Here's how the part is built. I have some questions about the finished solid (model axes, mm). Face numbers are marked on the shaded views. A direction names the side the tool comes from. Round coordinates to 2 decimals unless told otherwise and drop trailing zeros. Loops run counter-clockwise (first coordinate to the right, second up) from the corner with the lowest first, then second, coordinate; pieces in that order, holes last. Notation, with made-up numbers: M 74,42.5 L 98,42.5 A10 ccw 98,54.5 Z; hole C 0.25,-36.75 d8. An arc over 180 degrees is marked long. Use a Markdown table: item, result.
Autodesk Inventor part; units mm, degrees
ref_plane "Work Plane1" through (0, 0, -52.5) normal (0, 0, -1) x (-1, 0, 0)
ref_plane "YZ Plane" through (0, 0, 0) normal (1, 0, 0) x (0, 1, 0)
ref_plane "XZ Plane" through (0, 0, 0) normal (0, 1, 0) x (-1, 0, 0)
sketch "Sketch1" plane through (0, 0, 0) normal (0, 1, 0) x (-1, 0, 0)
  line L0 (0, 0) -> (105, 0)
  line L1 (105, 0) -> (105, -105)
  line L2 (105, -105) -> (0, -105)
  line L3 (0, -105) -> (0, 0)
  circle A0 centre (52.5, -52.5) radius 36.5
  dimension "d0" = 105
  dimension "d1" = 105
  dimension "d2" = 52.5
  dimension "d3" = 52.5
  dimension "d4" = 73
extrude "Extrusion1" add sketch "Sketch1" along normal blind 7
sketch "Sketch3" plane through (-105, 0, 0) normal (0, 0, 1) x (1, 0, 0)
  line L0 (105, 7) -> (0, 7)
  line L1 (0, 7) -> (105, 7)
  line L2 (105, 7) -> (105, -105)
  line L3 (105, -105) -> (0, -105)
  line L4 (0, -105) -> (0, 7)
  line L5 (0, 0) -> (105, 0)
  dimension "d7" = 105
extrude "Extrusion2" add sketch "Sketch3" along normal blind 5
sketch "Sketch4" plane through (-105, 0, -105) normal (-1, 0, 0) x (0, 0, 1)
  line L0 (0, 0) -> (0, 7)
  line L1 (0, 7) -> (110, 7)
  line L2 (110, 7) -> (110, -105)
  line L3 (110, -105) -> (0, -105)
  line L4 (0, -105) -> (0, 7)
  point P0 (105, 0)
extrude "Extrusion3" add sketch "Sketch4" along normal blind 5
sketch "Sketch6" plane through (0, 0, -105) normal (0, 0, -1) x (-1, 0, 0)
  line L0 (0, 7) -> (110, 7)
  line L1 (110, -105) -> (110, 7)
  line L2 (0, 7) -> (110, 7)
  line L3 (110, 7) -> (110, -105)
  line L4 (110, -105) -> (0, -105)
  line L5 (0, -105) -> (0, 7)
  point P0 (0, 0)
extrude "Extrusion4" add sketch "Sketch6" along normal blind 5
sketch "Sketch7" plane through (0, -105, 0) normal (1, 0, 0) x (0, 0, -1)
  line L0 (-5, 0) -> (-5, 112)
  line L1 (105, 0) -> (110, 0)
  line L2 (-5, 112) -> (110, 112)
  line L3 (110, 112) -> (110, 0)
  line L4 (110, 0) -> (-5, 0)
  line L5 (-5, 0) -> (-5, 112)
  point P0 (0, 105)
extrude "Extrusion5" add sketch "Sketch7" along normal blind 5
sketch "Sketch8" plane through (-110, -105, -110) normal (0, -1, 0) x (1, 0, 0)
  line L0 (0, 115) -> (115, 115)
  line L1 (0, 0) -> (115, 0)
  line L2 (0, 115) -> (115, 115)
  line L3 (115, 115) -> (115, 0)
  line L4 (115, 0) -> (0, 0)
  line L5 (0, 0) -> (0, 115)
  point P0 (110, 110)
extrude "Extrusion6" add sketch "Sketch8" along normal blind 5
sketch "Sketch9" plane through (0, 7, 0) normal (0, 1, 0) x (1, 0, 0)
  line L0 (-110, -5) -> (-110, 110)
  line L1 (-110, -5) -> (5, -5)
  line L2 (5, 110) -> (5, -5)
  line L3 (-110, 110) -> (5, 110)
  circle A0 centre (-52.5, 52.5) radius 36.5
  line L4 (-110, -5) -> (-110, 110)
  line L5 (-110, 110) -> (5, 110)
  line L6 (-110, -5) -> (5, -5)
  line L7 (5, -5) -> (5, 110)
  line L8 (5, 110) -> (-110, 110)
  line L9 (-110, 110) -> (-110, -5)
  circle A1 centre (-52.5, 52.5) radius 45
  dimension "d18" = 90
extrude "Extrusion7" add sketch "Sketch9" along normal blind 8 contours L0 L3 L2 L1
sketch "Sketch10" plane through (-52.5, 7, -52.5) normal (0, 1, 0) x (1, 0, 0)
  line L0 (57.5, -57.5) -> (-57.5, -57.5) construction
  line L1 (57.5, 57.5) -> (57.5, -57.5) construction
  line L2 (-57.5, -57.5) -> (57.5, 57.5) construction
  line L3 (57.5, 57.5) -> (-57.5, 57.5) construction
  line L4 (-57.5, 57.5) -> (57.5, -57.5) construction
  circle A0 centre (0, 0) radius 41.75 construction
  circle A1 centre (-29.5217, -29.5217) radius 1.9
  circle A2 centre (-29.5217, 29.5217) radius 1.9
  circle A3 centre (29.5217, 29.5217) radius 1.9
  circle A4 centre (29.5217, -29.5217) radius 1.9
  line L5 (0, -57.5) -> (0, 57.5) construction
  point P0 (52.5, -52.5)
  dimension "d21" = 3.8
  dimension "d22" = 83.5
  dimension "d23" = 3.8
  dimension "d24" = 3.8
  dimension "d25" = 3.8
  dimension "d26" = 45
extrude "Extrusion8" cut sketch "Sketch10" against normal blind 5
ref_plane "Work Plane1" through (0, 0, -52.5) normal (0, 0, -1) x (-1, 0, 0)
split "Split2" [suppressed]
chamfer "Chamfer1" distance 2 angle 45 1 edges at (-97.5, 15, -52.5)
sketch "Sketch15" plane through (0, 0, -52.5) normal (0, 0, -1) x (-1, 0, 0)
  line L0 (105, 14) -> (99.9142, 14)
  line L1 (99.9142, 14) -> (98.5, 12.5858)
  line L2 (98.5, 12.5858) -> (98.5, 6)
  line L3 (98.5, 6) -> (90, 6)
  line L4 (90, 6) -> (90, 1)
  line L5 (90, 1) -> (100, 1)
  arc A0 (106, -5) -> (100, 1) centre (100, -5) ccw
  line L6 (106, -5) -> (106, -100)
  arc A1 (100, -106) -> (106, -100) centre (100, -100) ccw
  line L7 (100, -106) -> (5, -106)
  arc A2 (-1, -100) -> (5, -106) centre (5, -100) ccw
  line L8 (-1, -100) -> (-1, -5)
  arc A3 (5, 1) -> (-1, -5) centre (5, -5) ccw
  line L9 (5, 1) -> (15, 1)
  line L10 (15, 1) -> (15, 6)
  line L11 (15, 6) -> (6.5, 6)
  line L12 (6.5, 6) -> (6.5, 12.5858)
  line L13 (6.5, 12.5858) -> (5.0858, 14)
  line L14 (5.0858, 14) -> (0, 14)
  arc A4 (0, 14) -> (-4, 10) centre (0, 10) ccw
  line L15 (-4, 10) -> (-4, -105)
  arc A5 (-4, -105) -> (0, -109) centre (0, -105) ccw
  line L16 (0, -109) -> (105, -109)
  arc A6 (105, -109) -> (109, -105) centre (105, -105) ccw
  line L17 (109, -105) -> (109, 10)
  arc A7 (109, 10) -> (105, 14) centre (105, 10) ccw
  line L18 (89, 0) -> (89, 7)
  line L19 (89, 7) -> (97.5, 7)
  line L20 (97.5, 7) -> (97.5, 13)
  line L21 (97.5, 13) -> (99.5, 15)
  line L22 (99.5, 15) -> (110, 15)
  line L23 (110, 15) -> (110, -110)
  line L24 (110, -110) -> (-5, -110)
  line L25 (-5, -110) -> (-5, 15)
  line L26 (-5, 15) -> (5.5, 15)
  line L27 (5.5, 15) -> (7.5, 13)
  line L28 (7.5, 13) -> (7.5, 7)
  line L29 (7.5, 7) -> (16, 7)
  line L30 (16, 7) -> (16, 0)
  line L31 (16, 0) -> (0, 0)
  line L32 (0, 0) -> (0, -105)
  line L33 (0, -105) -> (105, -105)
  line L34 (105, -105) -> (105, 0)
  line L35 (105, 0) -> (89, 0)
extrude "Extrusion11" [suppressed]
sketch "Sketch16" plane through (-110, -110, -110) normal (0, -1, 0) x (1, 0, 0)
  line L0 (10, 57.5) -> (105, 57.5)
  line L1 (10, 57.5) -> (10, 54.5)
  line L2 (10, 54.5) -> (105, 54.5)
  line L3 (105, 57.5) -> (105, 54.5)
  circle A0 centre (57.5, 56) radius 2
  line L4 (115, 57.5) -> (0, 57.5)
  point P0 (110, 110)
  point P1 (110, 57.5)
  point P2 (5, 57.5)
  dimension "d53" = 95
  dimension "d54" = 47.5
  dimension "d55" = 4
  dimension "d58" = 1.5
extrude "Extrusion14" [suppressed]
sketch "Sketch17" plane through (0, 0, -110) normal (0, 0, -1) x (-1, 0, 0)
  line L0 (110, 15) -> (110, -110)
  line L1 (110, -110) -> (-5, -110)
  line L2 (-5, -110) -> (-5, -160)
  line L3 (-5, -160) -> (110, -160)
  line L4 (110, -160) -> (110, -110)
  line L5 (-5, 15) -> (-5, -110)
  point P0 (0, 0)
  dimension "d59" = 50
extrude "Extrusion15" add sketch "Sketch17" against normal blind 5
sketch "Sketch18" plane through (5, -105, 0) normal (1, 0, 0) x (0, 0, -1)
  line L0 (105, -5) -> (-5, -5)
  line L1 (-5, -5) -> (-5, -55)
  line L2 (-5, -55) -> (105, -55)
  line L3 (105, -55) -> (105, -5)
  line L4 (-5, -5) -> (-5, 120)
  line L5 (110, -55) -> (105, -55)
  point P0 (0, 105)
extrude "Extrusion16" add sketch "Sketch18" against normal blind 5
sketch "Sketch19" plane through (-105, 0, 5) normal (0, 0, 1) x (1, 0, 0)
  line L0 (105, -110) -> (-5, -110)
  line L1 (-5, -160) -> (105, -160)
  line L2 (-5, -110) -> (105, -110)
  line L3 (105, -110) -> (105, -160)
  line L4 (105, -160) -> (-5, -160)
  line L5 (-5, -160) -> (-5, -110)
  point P0 (105, 0)
extrude "Extrusion17" add sketch "Sketch19" against normal blind 5
sketch "Sketch20" plane through (-110, 0, -105) normal (-1, 0, 0) x (0, 0, 1)
  line L0 (-5, -160) -> (110, -160)
  line L1 (0, -110) -> (105, -110)
  line L2 (105, -110) -> (105, -160)
  line L3 (105, -160) -> (0, -160)
  line L4 (0, -160) -> (0, -110)
  point P0 (105, 0)
extrude "Extrusion18" add sketch "Sketch20" against normal blind 5
sketch "Sketch21" plane through (-110, -160, -110) normal (0, -1, 0) x (1, 0, 0)
  line L0 (115, 0) -> (0, 0)
  line L1 (115, 115) -> (0, 115)
  line L2 (0, 0) -> (115, 0)
  line L3 (115, 0) -> (115, 115)
  line L4 (115, 115) -> (0, 115)
  line L5 (0, 115) -> (0, 0)
  point P0 (110, 110)
extrude "Extrusion19" add sketch "Sketch21" along normal blind 5
sketch "Sketch25" plane through (-110, -165, -110) normal (0, -1, 0) x (1, 0, 0)
  line L0 (65, 50) -> (105, 50) construction
  line L1 (105, 50) -> (105, 10) construction
  line L2 (105, 10) -> (65, 10) construction
  line L3 (65, 10) -> (65, 50) construction
  line L4 (65, 50) -> (105, 10) construction
  line L5 (105, 50) -> (65, 10) construction
  circle A0 centre (67, 46) radius 1.9
  circle A1 centre (103, 46) radius 1.9
  circle A2 centre (67, 25) radius 1.9
  circle A3 centre (103, 21) radius 1.9
  circle A4 centre (103, 46) radius 3.9
  circle A5 centre (67, 25) radius 3.9
  circle A6 centre (103, 21) radius 3.9
  line L6 (115, 0) -> (115, 115)
  line L7 (0, 0) -> (115, 0)
  line L8 (83, 14) -> (73, 14)
  line L9 (73, 14) -> (73, 29)
  line L10 (73, 29) -> (83, 29)
  line L11 (83, 29) -> (83, 14)
  line L12 (63, 50) -> (71, 50)
  line L13 (71, 50) -> (71, 42)
  line L14 (71, 42) -> (63, 42)
  line L15 (63, 42) -> (63, 50)
  line L16 (63, 50) -> (71, 42) construction
  line L17 (71, 50) -> (63, 42) construction
  point P0 (110, 110)
  point P1 (85, 30)
  dimension "d101" = 40
  dimension "d102" = 40
  dimension "d103" = 3.8
  dimension "d104" = 3.8
  dimension "d105" = 3.8
  dimension "d106" = 3.8
  dimension "d107" = 4
  dimension "d108" = 2
  dimension "d109" = 2
  dimension "d110" = 4
  dimension "d111" = 25
  dimension "d112" = 2
  dimension "d113" = 29
  dimension "d114" = 2
  dimension "d116" = 2
  dimension "d117" = 2
  dimension "d118" = 2
  dimension "d124" = 10
  dimension "d125" = 10
  dimension "d126" = 10
  dimension "d127" = 15
  dimension "d128" = 4
  dimension "d129" = 8
  dimension "d134" = 4
  dimension "d135" = 4
  dimension "d136" = 8
  dimension "d137" = 8
extrude "Extrusion23" add sketch "Sketch25" along normal blind 3 contours A4 | A5 | A6
extrude "Extrusion24" cut sketch "Sketch25" along normal blind 3 and the other way blind 5 contours L8 L9 L10 L11
sketch "Sketch26" plane through (0, 0, -110) normal (0, 0, -1) x (-1, 0, 0)
  line L0 (-5, 15) -> (-5, -165)
  line L1 (110, -165) -> (-5, -165)
  line L2 (105, -160) -> (0, -160) construction
  line L3 (40, -145) -> (0, -145)
  line L4 (0, -145) -> (0, -105)
  line L5 (0, -105) -> (40, -105)
  line L6 (40, -105) -> (40, -145)
  line L7 (33.4662, -145) -> (33.4662, -105) construction
  line L8 (3.4673, -145) -> (3.4673, -105) construction
  line L9 (40, -137.8014) -> (0, -137.8014) construction
  line L10 (0, -160) -> (0, -110) construction
  point P0 (0, 0)
  dimension "d142" = 40
  dimension "d143" = 40
  dimension "d144" = 20
  dimension "d145" = 5
equation "\"d2\" = 0.5 * d1"
equation "\"d3\" = 0.5 * d0"
equation "\"d23\" = d21"
equation "\"d24\" = d23"
equation "\"d25\" = d24"
equation "\"d54\" = 0.5 * d53"
equation "\"d104\" = d103"
equation "\"d105\" = d103"
equation "\"d106\" = d103"
equation "\"d112\" = d108"
equation "\"d114\" = d109"
equation "\"d116\" = d115"
equation "\"d117\" = d115"
equation "\"d118\" = d115"
properties part number "groovev2"
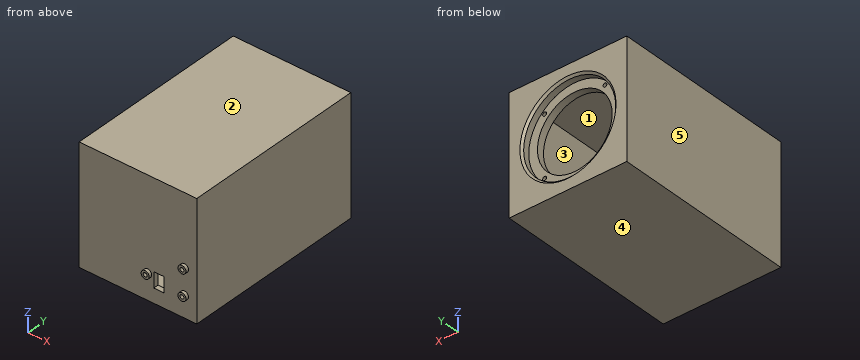
Q1. Imagine slicing it at D-D, the plane z = -13.5. Give the number of separate pieces and of enclosed holes in the cut face, then the cut area to 3 significant figures.
Return value:
| item | result |
|---|---|
| separate pieces | 1 |
| enclosed holes | 2 |
| area | 4,060 mm^2 |
Q2. Imagine slicing it at B-B, the plane y = -152. Please give me the cut outline in (x, z).
Return value:
| item | result |
|---|---|
| outline | M -110,-110 L 5,-110 L 5,5 L -110,5 Z; hole M -105,-105 L 0,-105 L 0,0 L -105,0 Z |
Q3. We'd pull the mould along Z, two halves only. Please class the marked faces 3, 4 and 5: pulls with the +Z half, pulls with the -Z half, needs draft (parallel to the pull), parting line crosses it, or undercut.
Return value:
| item | result |
|---|---|
| face 3 | undercut |
| face 4 | pulls with the -Z half |
| face 5 | needs draft |
Q4. Will these pins go through, and if not, where does the flat tip stop? P1, Ø1.9, axis at x = -7.5, z = -89.5, coming from the -Y side; P2, Ø2.5, axis at x = -22.98, z = -82.02, coming from the +Y side; P3, Ø5, axis at x = -45, z = -60.5, coming from the +Y side.
Return value:
| item | result |
|---|---|
| P1 | stops at y = -165 |
| P2 | stops at y = 2 |
| P3 | stops at y = -105 |
Q5. Imagine slicing it at C-C, the plane z = -52.5. Please give me the cut outline in (x, y).
Return value:
| item | result |
|---|---|
| outline | M -110,-165 L 5,-165 L 5,15 L -5.5,15 L -7.5,13 L -7.5,7 L -16,7 L -16,0 L 0,0 L 0,-105 L -105,-105 L -105,0 L -89,0 L -89,7 L -97.5,7 L -97.5,13 L -99.5,15 L -110,15 Z; hole M -105,-160 L 0,-160 L 0,-110 L -105,-110 Z |
Q6. Imagine slicing it at A-A, the plane x = -52.5. Please give me the cut outline in (y, z).
Return value:
| item | result |
|---|---|
| outline | M -165,-110 L 15,-110 L 15,-99.5 L 13,-97.5 L 7,-97.5 L 7,-89 L 0,-89 L 0,-105 L -105,-105 L -105,0 L 0,0 L 0,-16 L 7,-16 L 7,-7.5 L 13,-7.5 L 15,-5.5 L 15,5 L -165,5 Z; hole M -160,-105 L -110,-105 L -110,0 L -160,0 Z |
Q7. I need wall thicknesses on line 1 (Y direction, x = -102, z = -58); line 2 (Y direction, x = -25, z = -79); line 3 (X direction, y = -97.5, z = -27.5). Which ranges of each line are inside material? Lowest first, please. Write a range as from..to.
Return value:
| item | result |
|---|---|
| line 1 | y = -165..-160, -110..-105, 0..15 |
| line 2 | y = -165..-160, -110..-105, 0..7 |
| line 3 | x = -110..-105, 0..5 |
Q8. For the marked faces 1 and 2, which set-ups out of +Z, -Z, +X, -X, +Y, -Y let a thin tool reach every point of the face, with its end or its side?
Return value:
| item | result |
|---|---|
| face 1 | none |
| face 2 | +Z, +X, -X, +Y, -Y |
